Check sheet for the drawn part. Datum: minimum x, y, z corner. Units: mm. A direction names the side the tool comes from. Give positions to 0.01 mm unless a question says otherwise; leave off trailing zeros. Write each loop counter-clockwise with the first axis right and the second up, starting at its lowest first coordinate (ties: lowest second). Pieces come first, ordered by that corner, then holes.
(1) Thickness scan on line 1 along Y through (x, z) = (10.25, 5.5); line 2 along Z through (x, y) = (5.75, 19.75). Record the ranges inside material, lowest first.
(2) Depth check by flat-ended pin: P1, Ø2, axis at y = 12.5, z = 3.5, coming from the +X side; P2, Ø0.5, axis at x = 19.5, z = 1, coming from the -Y side; P3, Ø0.5, axis at x = 19.5, z = 1, coming from the +Y side. Enter the tip coordinate at first touch or a pass-through.
(3) Tool access check on the marked faces 1, 2 and 3. Record the directions out of +Z, -Z, +X, -X, +Y, -Y that give a thin tool (end or side, any length) a straight path to the whole face; none if there is none.
(4) Cross-section at B-B (y = 10.5). Record the boundary of the cut face in (x, z).
(5) Cross-section at C-C (z = 5). Record the boundary of the cut face in (x, y).
(6) Cross-section at A-A (z = 1). Record the boundary of the cut face in (x, y).
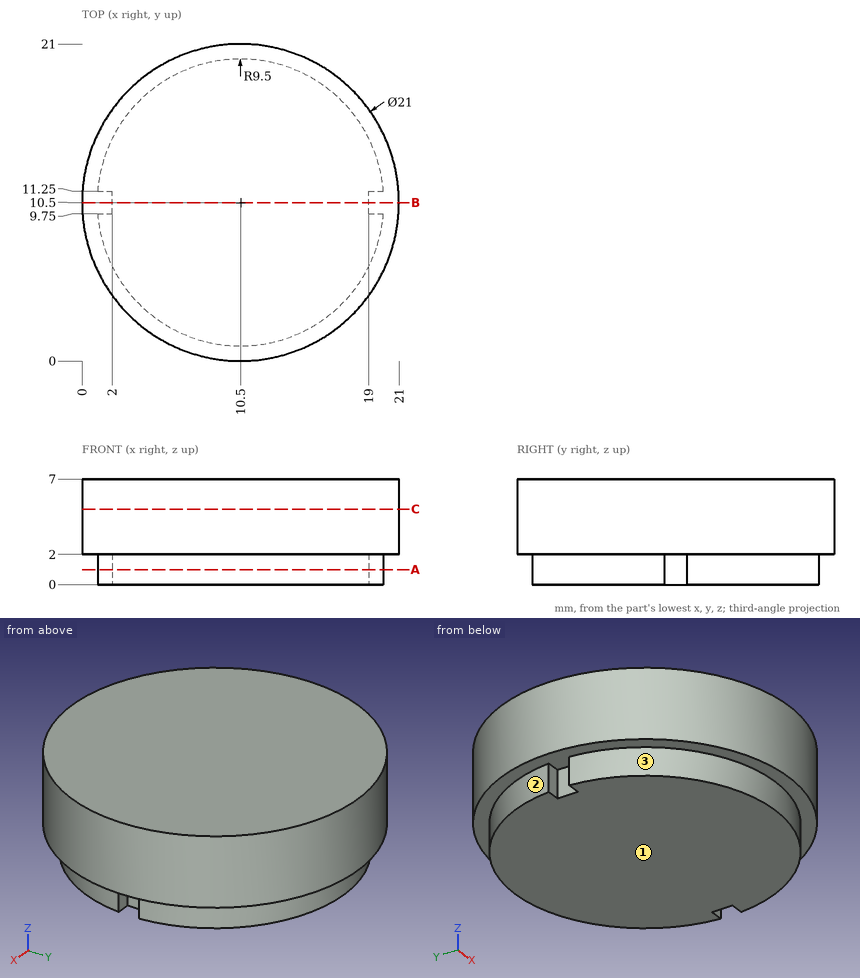
Reply:
1. line 1: y = 0 to 21
1. line 2: z = 2 to 7
2. P1: stops at x = 20.95
2. P2: stops at y = 6.8
2. P3: stops at y = 14.2
3. face 1: -Z, +X, -X, +Y, -Y
3. face 2: -Z, +Y
3. face 3: -Z, -Y
4. outline: (0, 2) - (2, 2) - (2, 0) - (19, 0) - (19, 2) - (21, 2) - (21, 7) - (0, 7) - close
5. outline: circle Ø21 at (10.5, 10.5)
6. outline: (1.03, 9.75) arc R9.5 ccw to (19.97, 9.75) - (19, 9.75) - (19, 11.25) - (19.97, 11.25) arc R9.5 ccw to (1.03, 11.25) - (2, 11.25) - (2, 9.75) - close
